```python
from build123d import *

# Parameters (mm, degrees)
CIRPATTERN1_COUNT = 3


with BuildPart() as part:
    # Sketch1 → Base-Revolve (revolve)
    with BuildSketch(Plane.XY):
        with BuildLine():
            Line((-100, 0), (-100, 1.25))
            ThreePointArc((-100, 1.25), (-99.010050505, 7.072345027), (-96.68190465, 12.5))
            Line((-96.68190465, 12.5), (-3.349364905, 12.5))
            ThreePointArc((-3.349364905, 12.5), (-0.851854343, 6.470476128), (0, 0))
            Line((0, 0), (-100, 0))
        make_face()
    revolve(axis=Axis((-40, 0, 0), (1, 0, 0)))

    # Cut-Sweep1: sweep along a path in Sketch4
    with BuildLine(Plane(origin=(0, 0, 0), x_dir=(1, 0, 0), z_dir=(0, 1, 0))) as cut_sweep1_path:
        Line((0, -11.25), (-100, -12.5))
    # Sketch2 → Cut-Sweep1 (sweep, cut)
    with BuildSketch(Plane(origin=(0, 0, 0), x_dir=(0, 0, -1), z_dir=(1, 0, 0))):
        Polygon((-11.25, 0), (-12.5, 0.875259423), (-12.5, -0.875259423), align=None)
    cut_sweep1 = sweep(path=cut_sweep1_path.line, mode=Mode.SUBTRACT)

    # CirPattern1: Cut-Sweep1 ×3 about axis
    cirpattern1_axis = Axis((0, 0, 0), (1, 0, 0))
    for i in range(1, CIRPATTERN1_COUNT):
        add(cut_sweep1.rotate(cirpattern1_axis, i * 360 / CIRPATTERN1_COUNT), mode=Mode.SUBTRACT)


solid = part.part
```
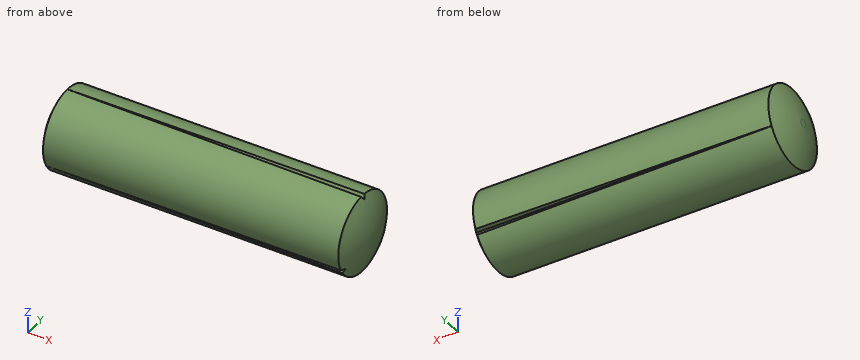
Verification items for the finished model (mm, model axes). Round coordinates to 2 decimals unless told otherwise and drop trailing zeros. Order: outer loops, then holes, each group sorted by start corner. A loop starts at its lowest first (then second) coordinate and runs counter-clockwise, first axis right, second up. Notation, with made-up numbers: (-8.75, 54) - (-2.75, 54) arc R6 ccw to (-2.75, 65) - close; hole circle Ø7 at (16.5, 30). An arc over 180 degrees is marked (long way). Use CSV: the item, a comma, the result in double quotes. Start each with the question number.
1) Section check C-C, the plane y = -2.75. Record the cut outline in (x, z), plus the area to 3 significant figures.
2) Section check A-A, the plane x = -6.5. Record the cut outline in (y, z).
3) Section check D-D, the plane x = -19.5. Record the cut outline in (y, z).
4) Go/stop test with flat-tipped pins: P1, Ø1.5, axis at x = -82, y = 2.5, coming from the +Z side; P2, Ø10, axis at x = -34, y = -3.5, coming from the +Z side; P3, Ø4, axis at x = -64.5, z = -9, coming from the -Y side. Record where each tip stops, or that it passes through.
5) Section check B-B, the plane z = -3.5. Record the cut outline in (x, y).
6) Thickness scan on L1, parallel to Z at x = -46, y = 6.25; L2, parallel to Z at x = -17, y = 0.75; L3, parallel to Y at x = -9.5, z = 5. Record the ranges inside material, lowest first.
Answers:
1,outline,"(-96.68, -12.19) - (-3.35, -12.19) arc R24.85 ccw to (-3.35, 12.19) - (-96.68, 12.19) arc R24.85 ccw to start"
1,area,"2,380 mm²"
2,outline,"(-11.2, -5.54) - (-9.81, -5.67) - (-10.4, -6.93) arc R12.5 ccw to (10.4, -6.93) - (9.81, -5.67) - (11.2, -5.54) arc R12.5 ccw to (0.8, 12.47) - (0, 11.33) - (-0.8, 12.47) arc R12.5 ccw to start"
3,outline,"(-11.15, -5.64) - (-9.95, -5.75) - (-10.46, -6.84) arc R12.5 ccw to (10.46, -6.84) - (9.95, -5.75) - (11.15, -5.64) arc R12.5 ccw to (0.69, 12.48) - (0, 11.49) - (-0.69, 12.48) arc R12.5 ccw to start"
4,P1,"stops at z = 12.38"
4,P2,"stops at z = 12.49"
4,P3,"stops at y = -10.36"
5,outline,"(-96.68, -12) - (-3.35, -12) arc R24.75 ccw to (-3.35, 12) - (-96.68, 12) arc R24.75 ccw to start"
6,L1,"z = -10.83 to 10.83"
6,L2,"z = -12.48 to 12.48"
6,L3,"y = -11.46 to 11.46"
